Geometry check sheet. Reference: drawing and pictorial views, mm from the part's lowest x, y, z. Round coordinates to 2 decimals unless told otherwise and drop trailing zeros. Loops run counter-clockwise (first coordinate to the right, second up) from the corner with the lowest first, then second, coordinate; pieces in that order, holes last. Notation, with made-up numbers: (85, -5) - (110, -5) arc R32 ccw to (110, 31) - close; hole circle Ø11 at (87, -7). An arc over 180 degrees is marked (long way). Return JSON: item names as keys, results as strings.
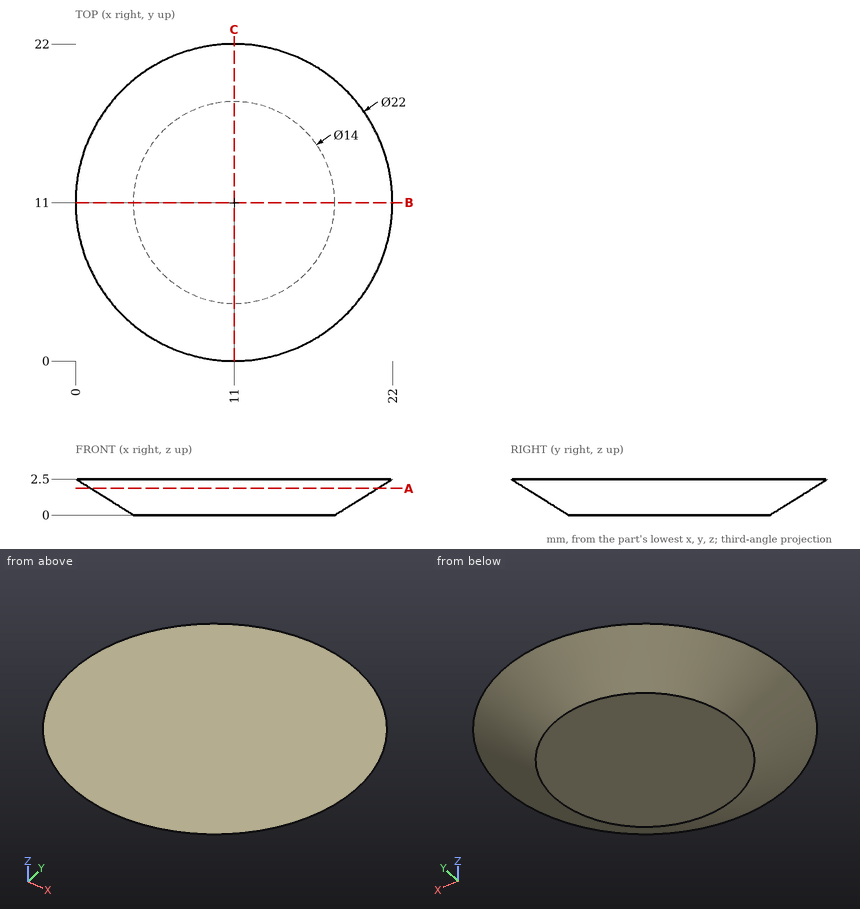
Q1. Scan lines: probe 1 along Z at (x, y) = (3.25, 12.5); probe 2 along Y at (x, z) = (5, 1.45); probe 3 along Z at (x, y) = (4.75, 4.5). Record each from-to range of solid material in increasing order. Write a range as [from, to].
Answer key:
{"probe 1": "z = [0.56, 2.5]", "probe 2": "y = [3.87, 18.13]", "probe 3": "z = [1.26, 2.5]"}
Q2. Sectioned sample at A-A (z = 1.85). Enter the section's corners in (x, y).
Answer key:
{"outline": "circle Ø19.92 at (11, 11)"}
Q3. Depth check by flat-ended pin: P1, Ø1.5, axis at x = 12.5, z = 1.5, coming from the -Y side; P2, Ø1, axis at y = 16, z = 2, coming from the +X side. Enter the tip coordinate at first touch or a pass-through.
Answer key:
{"P1": "stops at y = 0.5", "P2": "stops at x = 20.83"}
Q4. Sectioned sample at B-B (y = 11). Enter the section's corners in (x, z).
Answer key:
{"outline": "(0, 2.5) - (4, 0) - (18, 0) - (22, 2.5) - close"}
